Work out the finished part from the listing and answer in its coordinate system (mm). Face numbers are marked on the shaded views. A direction names the side the tool comes from. Round coordinates to 2 decimals unless told otherwise and drop trailing zeros. Loops run counter-clockwise (first coordinate to the right, second up) from the corner with the lowest first, then second, coordinate; pieces in that order, holes last. Notation, with made-up numbers: (-31, 30.25) -> (3, 30.25) arc R27 cw to (3, 63.25) -> close; hole circle Ø4 at (-35, 46). An arc over 180 degrees is marked (long way). Use one line per item in the form item = value.
```python
from build123d import *

# Parameters (mm, degrees)
SKETCH1_W               = 30
SKETCH1_H               = 30
BOSS_EXTRUDE1_DEPTH     = 3
SKETCH3_W               = 30
SKETCH3_H               = 30
BOSS_EXTRUDE2_DEPTH     = 3
SKETCH4_W               = 30
SKETCH4_H               = 10
BOSS_EXTRUDE3_DEPTH     = 4
CUT_EXTRUDE1_DEPTH      = 48.602520942
CUT_EXTRUDE1_DEPTH_BACK = 48.602520942
SKETCH2_R               = 1.4
SKETCH2_R_2             = 0.9
FILLET1_R               = 4
FILLET2_R               = 2


with BuildPart() as part:
    # Sketch1 → Boss-Extrude1 (new body)
    with BuildSketch(Plane(origin=(0, 0, 0), x_dir=(1, 0, 0), z_dir=(0, 1, 0))):
        Rectangle(SKETCH1_W, SKETCH1_H)
    extrude(amount=BOSS_EXTRUDE1_DEPTH)

    # Sketch3 → Boss-Extrude2 (add)
    with BuildSketch(Plane(origin=(0, 3, 0), x_dir=(1, 0, 0), z_dir=(0, 1, 0))):
        with Locations((0, 30)):
            Rectangle(SKETCH3_W, SKETCH3_H)
    extrude(amount=-BOSS_EXTRUDE2_DEPTH)

    # Sketch4 → Boss-Extrude3 (add)
    with BuildSketch(Plane(origin=(0, 3, 0), x_dir=(1, 0, 0), z_dir=(0, 1, 0))):
        with Locations((0, -10)):
            Rectangle(SKETCH4_W, SKETCH4_H)
        with Locations((0, 26)):
            Rectangle(SKETCH4_W, SKETCH4_H)
    extrude(amount=BOSS_EXTRUDE3_DEPTH)

    # Sketch2 → Cut-Extrude1 (cut, two sides: drawn at the far end of the back side and taken through both)
    with BuildSketch(Plane(origin=(0, 3, 0), x_dir=(1, 0, 0), z_dir=(0, 1, 0)).offset(-CUT_EXTRUDE1_DEPTH_BACK)):
        with Locations(Location((-10, -10, 0), (0, 0, 270))):
            Circle(SKETCH2_R)
        with Locations(Location((10, -10, 0), (0, 0, 270))):
            Circle(SKETCH2_R)
        with Locations(Location((10, 10, 0), (0, 0, 90))):
            Circle(SKETCH2_R)
        with Locations(Location((-10, 10, 0), (0, 0, 90))):
            Circle(SKETCH2_R)
        with Locations(Location((-10.795, 33.24, 0), (0, 0, 90))):
            Circle(SKETCH2_R_2)
        with Locations(Location((10.795, 33.24, 0), (0, 0, 90))):
            Circle(SKETCH2_R_2)
        with Locations(Location((10.795, 18, 0), (0, 0, 90))):
            Circle(SKETCH2_R_2)
        with Locations(Location((-10.795, 18, 0), (0, 0, 90))):
            Circle(SKETCH2_R_2)
        with Locations(Location((-10.795, 41.24, 0), (0, 0, 90))):
            Circle(SKETCH2_R_2)
        with Locations(Location((10.795, 41.24, 0), (0, 0, 90))):
            Circle(SKETCH2_R_2)
        with BuildLine():
            Line((-3, -9), (3, -9))
            ThreePointArc((3, -9), (7.242640687, -7.242640687), (9, -3))
            Line((9, -3), (9, 3))
            ThreePointArc((9, 3), (7.242640687, 7.242640687), (3, 9))
            Line((3, 9), (-3, 9))
            ThreePointArc((-3, 9), (-7.242640687, 7.242640687), (-9, 3))
            Line((-9, 3), (-9, -3))
            ThreePointArc((-9, -3), (-7.242640687, -7.242640687), (-3, -9))
        make_face()
        with BuildLine():
            Line((-5, 19.267058824), (5, 19.267058824))
            ThreePointArc((5, 19.267058824), (7.828427125, 20.438631699), (9, 23.267058824))
            Line((9, 23.267058824), (9, 27.972941176))
            ThreePointArc((9, 27.972941176), (7.828427125, 30.801368301), (5, 31.972941176))
            Line((5, 31.972941176), (-5, 31.972941176))
            ThreePointArc((-5, 31.972941176), (-7.828427125, 30.801368301), (-9, 27.972941176))
            Line((-9, 27.972941176), (-9, 23.267058824))
            ThreePointArc((-9, 23.267058824), (-7.828427125, 20.438631699), (-5, 19.267058824))
        make_face()
    extrude(amount=CUT_EXTRUDE1_DEPTH + CUT_EXTRUDE1_DEPTH_BACK, mode=Mode.SUBTRACT)

    # Fillet1
    fillet1_edges = [part.edges().sort_by_distance(p)[0] for p in [
        (-15, 1.5, -45),
        (15, 1.5, -45),
        (15, 3.5, 15),
        (-15, 3.5, 15),
        (15, 5, 5),
        (8.656854249, 5, 5),
        (-8.656854249, 5, 5),
        (-15, 5, 5),
        (15, 5, -21),
        (15, 5, -31),
        (-15, 5, -21),
        (-15, 5, -31),
    ]]
    fillet(fillet1_edges, radius=FILLET1_R - 0.0001)  # a hair under: the kernel refuses the full size

    # Fillet2
    fillet2_edges = [part.edges().sort_by_distance(p)[0] for p in [
        (-8.29551882, 5, -21),
        (8.29551882, 5, -21),
        (7.614749487, 5, -31),
        (-7.614749487, 5, -31),
    ]]
    fillet(fillet2_edges, radius=FILLET2_R)


solid = part.part
```
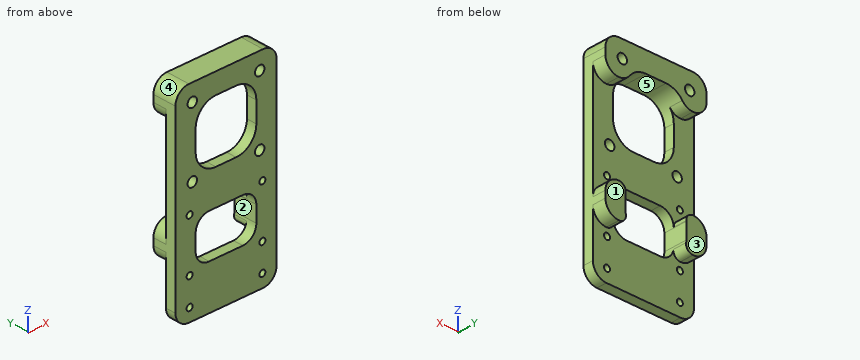
(1) Consider L1, parallel to X at y = 0.7, z = -18 (3 decimals); L2, parallel to X at y = 3.75, z = 10; L3, parallel to Z at x = 6.75, y = 0.5. Determine where each line is inside the solid, lowest interval first.
Completed:
L1 = -15 to -11.695, -9.895 to 9.895, 11.695 to 15
L2 = -15 to -11.4, -8.6 to 8.6, 11.4 to 15
L3 = -45 to -31.57, -19.67 to -7.68, 7.68 to 15
(2) Find section C-C, the plane z = -24. Write down the section's boundary in (x, y).
Completed:
outline = (-15, 0) -> (-9, 0) -> (-9, 7) -> (-14.87, 7) -> (-14.87, 3) -> (-15, 3) -> close; (9, 0) -> (15, 0) -> (15, 3) -> (14.87, 3) -> (14.87, 7) -> (9, 7) -> close
(3) For the marked faces 1 and 2, determine the directions among +Z, -Z, +X, -X, +Y, -Y from which every point of the face is accessible in a straight line to the end or side of a thin tool.
Completed:
face_1 = +Z, -Z, +X, -X, +Y
face_2 = +Y, -Y
(4) Find section D-D, the plane y = 1.5. State how many separate pieces and enclosed holes the cut face has, then the cut area to 3 significant figures.
Completed:
separate_pieces = 1
enclosed_holes = 12
area = 1,240 mm2
(5) Given P1, Ø2, axis at y = 4.5, z = -3.5, coming from the -X side; P2, Ø2, axis at x = -9, z = -31.5, coming from the +Y side; P3, Ø2, axis at y = 4.5, z = 4.5, coming from the +X side, each flat-ended and moving along its own axis, determine where each tip first touches the part or whether it passes through.
Completed:
P1 = through
P2 = 3
P3 = 12.94
(6) Find section A-A, the plane x = -2.25. Write down the section's boundary in (y, z), then the cut area to 3 significant figures.
Completed:
outline = (0, -45) -> (3, -45) -> (3, -31.97) -> (0, -31.97) -> close; (0, -19.27) -> (3, -19.27) -> (3, -9) -> (0, -9) -> close; (0, 9) -> (7, 9) -> (7, 15) -> (0, 15) -> close
area = 112 mm2
(7) Find section B-B, the plane z = -10. Write down the section's boundary in (x, y).
Completed:
outline = (-15, 0) -> (-11.4, 0) -> (-11.4, 3) -> (-15, 3) -> close; (-8.6, 0) -> (8.6, 0) -> (8.6, 3) -> (-8.6, 3) -> close; (11.4, 0) -> (15, 0) -> (15, 3) -> (11.4, 3) -> close
(8) For a pull along X with two mould halves and no side action, classify the marked faces 3, 4 and 5 as +X half, -X half, draft (parallel to the pull), parting line (faces both ways), or undercut.
Completed:
face_3 = draft
face_4 = -X half
face_5 = undercut
